The listing builds one solid part. Answer for the finished solid, in the listing's coordinates (mm). Give positions to 0.01 mm unless a question says otherwise; leave off trailing zeros. Order: outer loops, then holes, each group sorted by start corner. A loop starts at its lowest first (then second) coordinate and runs counter-clockwise, first axis right, second up.
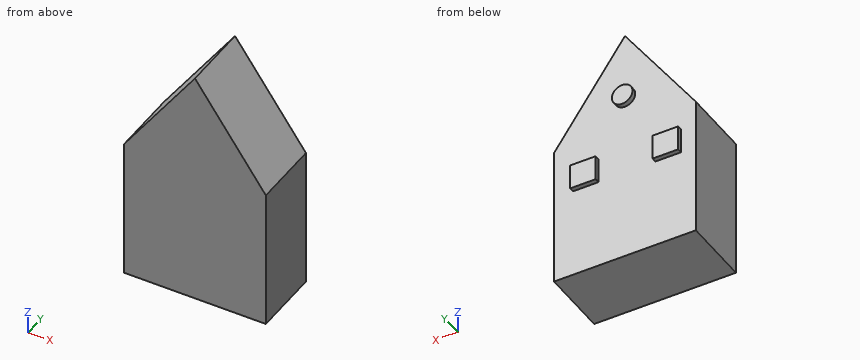
```python
from build123d import *

# Parameters (mm, degrees)
F0_W     = 52.538685
F0_H     = 52.353366
F2_DEPTH = 25.4
F1_W     = 9.434705
F1_H     = 9.342208
F1_W_2   = 9.434706
F1_R     = 3.813753
F3_DEPTH = 1.778


with BuildPart() as f2:
    # F0 (on Front) → F2 (new body)
    with BuildSketch(Plane.XZ):
        with Locations((0.000164, -7.769757)):
            Rectangle(F0_W, F0_H)
        Polygon((0.000164, 55.590764), (-26.269179, 18.406926), (26.269506, 18.406926), align=None)
    extrude(amount=F2_DEPTH)

    # F1 (on Front) → F3 (join)
    with BuildSketch(Plane.XZ):
        with Locations((-16.002, 4.671104)):
            Rectangle(F1_W, F1_H)
        with Locations((14.522046, 4.671104)):
            Rectangle(F1_W_2, F1_H)
        with Locations((0, 30.616544)):
            Circle(F1_R)
    extrude(amount=-F3_DEPTH)


solid = f2.part
```
1) Find section C-C (z = -15). Write down the section's boundary in (x, y).
Geometry says:
outline: (-26.27, -25.4) - (26.27, -25.4) - (26.27, 0) - (-26.27, 0) - close
2) Straight lines are drawn through the part: probe 1 along Y at (x, z) = (-3, 18.5); probe 2 along X at (y, z) = (-15.25, 26); probe 3 along Z at (x, y) = (-23, -15.25). For each, find the intervals that lie inside material, in ascending order.
Geometry says:
probe 1: y = -25.4 to 0
probe 2: x = -20.9 to 20.91
probe 3: z = -33.95 to 23.03
3) Find section D-D (x = 12.5). Write down the section's boundary in (y, z).
Geometry says:
outline: (-25.4, -33.95) - (0, -33.95) - (0, 0) - (1.78, 0) - (1.78, 9.34) - (0, 9.34) - (0, 37.9) - (-25.4, 37.9) - close
4) Find section A-A (x = -14.5). Write down the section's boundary in (y, z), then the cut area to 3 significant figures.
Geometry says:
outline: (-25.4, -33.95) - (0, -33.95) - (0, 0) - (1.78, 0) - (1.78, 9.34) - (0, 9.34) - (0, 35.07) - (-25.4, 35.07) - close
area: 1,770 mm2
5) Given P1, Ø0.9, axis at y = 1, z = 2.5, coming from the -X side; P2, Ø8, axis at x = -18.5, y = -15.5, coming from the +Z side; P3, Ø8, axis at x = 15.5, y = -21, coming from the +Z side; P4, Ø2, axis at x = 16.5, y = 0.5, coming from the -Z side, each flat-ended and moving along its own axis, determine where each tip first touches the part or whether it passes through.
Geometry says:
P1: stops at x = -20.72
P2: stops at z = 35.07
P3: stops at z = 39.31
P4: stops at z = -33.95
6) Find section B-B (y = -13.75). Write down the section's boundary in (x, z).
Geometry says:
outline: (-26.27, -33.95) - (26.27, -33.95) - (26.27, 18.41) - (0, 55.59) - (-26.27, 18.41) - close
